For this review, use the dimensioned drawing (mm, ordinates from the lowest corner) and the shaded views. Give positions to 0.01 mm unless a question says otherwise; leave off trailing zeros. Write each loop counter-clockwise with the first axis right and the second up, starting at its lowest first coordinate (ties: lowest second). Pieces come first, ordered by that corner, then holes. Notation, with made-up numbers: (20, 69) -> (79, 69) arc R25 cw to (79, 89) -> close; hole circle Ø7 at (-16.5, 22). An arc over 180 degrees is marked (long way). Return JSON: item names as keys, results as strings.
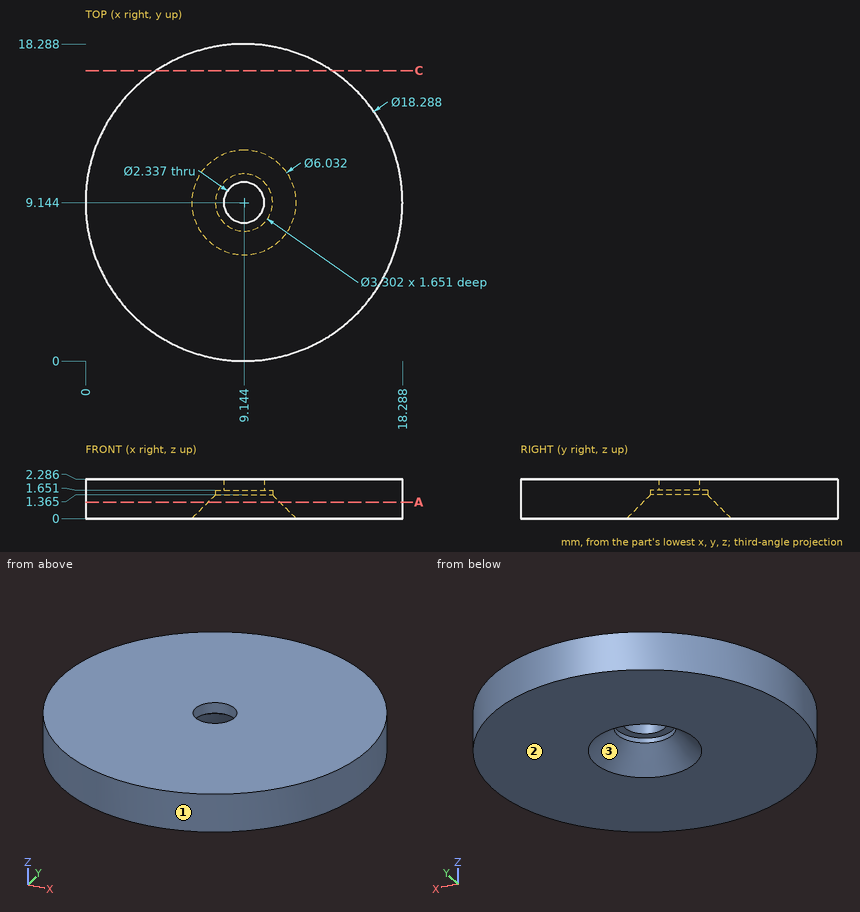
1. The part is to be moulded in two halves that separate along Y. For the marked faces 1, 2 and 3, say which applies: +Y half, -Y half, draft (parallel to the pull), parting line (faces both ways), or undercut.
Results found:
{"face 1": "parting line", "face 2": "draft", "face 3": "undercut"}
2. Add section C-C, the plane y = 16.75. State the section outline as (x, z) points (1 decimal).
Results found:
{"outline": "(4.1, 0) -> (14.2, 0) -> (14.2, 2.3) -> (4.1, 2.3) -> close"}
3. For pin 1 (1.7 mm diameter, centred on x = 9, y = 9.5, fed in from -Z); pin 2 (1.4 mm diameter, centred on x = 9.144, y = 9.144, fed in from -Z), all flat-tipped, find the tip position at first contact; note any pin that passes through.
Results found:
{"pin 1": "stops at z = 1.65", "pin 2": "passes through"}
4. To check wall thickness, follow probe 1 along X at (y, z) = (9, 0.55) (1 decimal); probe 2 along Y at (x, z) = (5, 2) (1 decimal); probe 3 along Y at (x, z) = (15, 0.2) (1 decimal). State the ranges of each line that lie inside material, in increasing order.
Results found:
{"probe 1": "x = 0 to 6.7, 11.6 to 18.3", "probe 2": "y = 1 to 17.3", "probe 3": "y = 2.1 to 16.2"}
5. Add section A-A, the plane z = 0.95. State the section outline as (x, y) points (1 decimal), plus the area to 3 significant figures.
Results found:
{"outline": "circle Ø18.3 at (9.1, 9.1); hole circle Ø4.1 at (9.1, 9.1)", "area": "249 mm²"}
